from build123d import *

# Parameters (mm, degrees)
SKETCH1_R           = 50.8
SKETCH1_R_2         = 2.2225
SKETCH1_R_3         = 4.0132
BOSS_EXTRUDE1_DEPTH = 19.05


with BuildPart() as part:
    # Sketch1 → Boss-Extrude1 (new body)
    with BuildSketch(Plane(origin=(0, 0, 0), x_dir=(1, 0, 0), z_dir=(0, 1, 0))):
        Circle(SKETCH1_R)
        Circle(SKETCH1_R_2, mode=Mode.SUBTRACT)
        with BuildLine():
            add(Edge.make_bspline(
                [(47.425, 8.028719366), (47.425, 21.375976625), (33.958540857, 19.868664087), (20.492081715, 18.361351549), (23.533629849, 5.35453743)],
                knots=[0, 0, 0, 1.683968262, 1.683968262, 3.367936524, 3.367936524, 3.367936524], degree=2, weights=[1, 0.665984043, 1, 0.665984043, 1]))
            add(Edge.make_bspline(
                [(47.116370151, 5.35453743), (47.425, 6.674355793), (47.425, 8.028719366)],
                knots=[6.056841437, 6.056841437, 6.056841437, 6.283185307, 6.283185307, 6.283185307], degree=2, weights=[1, 0.993602889, 1]))
            add(Edge.make_bspline(
                [(44.525, -5.059632012), (48.484325385, -0.495358305), (47.116370151, 5.35453743)],
                knots=[5.576210889, 5.576210889, 5.576210889, 6.500952743, 6.500952743, 6.500952743], degree=2, weights=[1, 0.843252924, 0.891535306]))
            add(Edge.make_bspline(
                [(23.533629849, 5.35453743), (23.225, 4.034719066), (23.225, 2.680355494), (23.225, -29.614075135), (44.525, -5.059632012)],
                knots=[2.868291657, 2.868291657, 2.868291657, 3.141592654, 3.141592654, 5.576210889, 5.576210889, 5.576210889], degree=2, weights=[0.869685773, 0.926603696, 1, 0.346171505, 1]))
        make_face(mode=Mode.SUBTRACT)
        with Locations((1.27, 41.91)):
            Circle(SKETCH1_R_3, mode=Mode.SUBTRACT)
    extrude(amount=BOSS_EXTRUDE1_DEPTH)


solid = part.part
Can you work these out from the model? Positions are in its coordinate system, mm. Coordinates: 2 decimals unless noted, no trailing zeros. Loops run counter-clockwise (first coordinate to the right, second up) from the corner with the lowest first, then second, coordinate; pieces in that order, holes last. Notation, with made-up numbers: M 86,25 L 120,25 A34 ccw 120,55 Z; hole C 58,-7.5 d8. An arc over 180 degrees is marked long. Return JSON: item names as keys, results as strings. Group by question number.
Item 1: Imagine slicing it at B-B (z = 0). Give the number of separate pieces and of enclosed holes in the cut face, and give its area (3 significant figures).
Item 2: Imagine slicing it at C-C (x = 9). Please give me the cut outline in (y, z), and give its area (3 significant figures).
Item 3: I'm going to push flat-ended pins straight in: pin 1 Ø1.5 at (x, z) = (-11.5, -31) entering from -Y; pin 2 Ø5 at (x, z) = (1.27, -41.91) entering from -Y; pin 3 Ø3 at (y, z) = (10, 29) entering from -X; pin 4 Ø3 at (y, z) = (16.5, -21) entering from -X. Where does each tip first touch, or does it pass through?
Item 4: Imagine slicing it at A-A (z = -41.91). Please give me the cut outline in (x, y).
Item 5: Thinking about a two-plate mould opening in Z: for faces 1 (the cylindrical face through (0.4, 9.392, -37.992)), 2 (the cylindrical face through (-0.48, 9.39, 2.17)), 3 (the flat face through (-1, 0, 11)), 4 (the cylindrical face through (-11.012, 9.392, 49.592)), which applies, released by +Z, released by -Z, zero draft, split by the parting line, or undercut?
Item 6: If I drill on L1, parallel to Z at x = 0, y = 11.25; L2, parallel to Z at x = 1.27, y = 12; L3, parallel to X at y = 13, z = -1, over which ranges is the centre line in solid material (lowest first)? Write a range as from..to.
Verdict:
{
 "1": {"separate pieces": "3", "enclosed holes": "0", "area": "1,400 mm^2"},
 "2": {"outline": "M 0,-50 L 19.05,-50 L 19.05,50 L 0,50 Z", "area": "1,900 mm^2"},
 "3": {"pin 1": "stops at y = 0", "pin 2": "passes through", "pin 3": "stops at x = -42.71", "pin 4": "stops at x = -46.91"},
 "4": {"outline": "M -28.71,0 L -2.74,0 L -2.74,19.05 L -28.71,19.05 Z; M 5.28,0 L 28.71,0 L 28.71,19.05 L 5.28,19.05 Z"},
 "5": {"face 1": "undercut", "face 2": "undercut", "face 3": "zero draft", "face 4": "split by the parting line"},
 "6": {"L1": "z = -50.8..-45.72, -38.1..-2.22, 2.22..50.8", "L2": "z = -50.78..-45.92, -37.9..-1.82, 1.82..50.78", "L3": "x = -50.79..-1.98, 1.98..23.35, 47.3..50.79"}
}
